```python
from build123d import *

# Parameters (mm, degrees)
SKETCH1_R                    = 69.85
SKETCH1_R_2                  = 55.88
BOSS_EXTRUDE1_DEPTH          = 6.35
BOSS_EXTRUDE2_DEPTH          = 6.35
FILLET1_R                    = 6.35
CIRPATTERN2_COUNT            = 4
FILLET1_OF_CIRPATTERN2_R     = 6.35
F_0_257_DIAMETER_HOLE1_D     = 6.5278
CIRPATTERN1_COUNT            = 4
SKETCH6_R                    = 3.2639
CUT_EXTRUDE1_DEPTH           = 7.3500001
BOSS_EXTRUDE4_DEPTH          = 6.35
FILLET3_R                    = 3.175
F_18_0_1695_DIAMETER_HOLE1_D = 4.3053


with BuildPart() as part:
    # Sketch1 → Boss-Extrude1 (new body)
    with BuildSketch(Plane(origin=(0, 0, 0), x_dir=(1, 0, 0), z_dir=(0, 1, 0))):
        Circle(SKETCH1_R)
        Circle(SKETCH1_R_2, mode=Mode.SUBTRACT)
    extrude(amount=BOSS_EXTRUDE1_DEPTH)

    # Sketch5 → Boss-Extrude2 (add)
    with BuildSketch(Plane(origin=(0, 6.35, 0), x_dir=(1, 0, 0), z_dir=(0, 1, 0))):
        with BuildLine():
            Line((-9.525, 63.5), (9.525, 63.5))
            Line((9.525, 63.5), (9.525, 73.025))
            ThreePointArc((9.525, 73.025), (7.665128061, 77.515128061), (3.175, 79.375))
            Line((3.175, 79.375), (-3.175, 79.375))
            ThreePointArc((-3.175, 79.375), (-7.665128061, 77.515128061), (-9.525, 73.025))
            Line((-9.525, 73.025), (-9.525, 63.5))
        make_face()
    boss_extrude2 = extrude(amount=-BOSS_EXTRUDE2_DEPTH)

    # Fillet1
    fillet1_edges = [part.edges().sort_by_distance(p)[0] for p in [
        (9.525, 3.175, -69.197520729),
        (-9.525, 3.175, -69.197520729),
    ]]
    fillet(fillet1_edges, radius=FILLET1_R)

    # CirPattern2: Boss-Extrude2 ×4 about axis
    cirpattern2_axis = Axis((0, 0, 0), (0, 1, 0))
    for i in range(1, CIRPATTERN2_COUNT):
        add(boss_extrude2.rotate(cirpattern2_axis, i * 360 / CIRPATTERN2_COUNT))

    # Fillet1 of CirPattern2
    fillet1_of_cirpattern2_edges = [part.edges().sort_by_distance(p)[0] for p in [
        (-69.197520729, 3.175, -9.525),
        (-69.197520729, 3.175, 9.525),
        (-9.525, 3.175, 69.197520729),
        (9.525, 3.175, 69.197520729),
        (69.197520729, 3.175, 9.525),
        (69.197520729, 3.175, -9.525),
    ]]
    fillet(fillet1_of_cirpattern2_edges, radius=FILLET1_OF_CIRPATTERN2_R)

    # F (0.257) Diameter Hole1 (through all)
    with Locations(Plane(origin=(0, 6.35, 0), x_dir=(1, 0, 0), z_dir=(0, 1, 0))):
        with Locations((69.85, 0)):
            f_0_257_diameter_hole1 = Hole(F_0_257_DIAMETER_HOLE1_D / 2)

    # CirPattern1: F (0.257) Diameter Hole1 ×4 about axis
    cirpattern1_axis = Axis((0, 0, 0), (0, 1, 0))
    for i in range(1, CIRPATTERN1_COUNT):
        add(f_0_257_diameter_hole1.rotate(cirpattern1_axis, i * 360 / CIRPATTERN1_COUNT), mode=Mode.SUBTRACT)

    # Sketch6 → Cut-Extrude1 (cut, through all)
    with BuildSketch(Plane.XZ):
        with BuildLine():
            Line((-38.749062578, -40.262694263), (-48.149496878, -50.60285022))
            ThreePointArc((-48.149496878, -50.60285022), (-46.98699519, -51.684086361), (-45.800220226, -52.738622728))
            Line((-45.800220226, -52.738622728), (-36.399785925, -42.398466772))
            ThreePointArc((-36.399785925, -42.398466772), (-37.589596152, -41.347269089), (-38.749062578, -40.262694263))
        make_face()
        with BuildLine():
            Line((-36.399785925, -42.398466772), (-45.800220226, -52.738622728))
            ThreePointArc((-45.800220226, -52.738622728), (-31.12686289, -62.531119506), (-14.468129908, -68.335171888))
            add(Edge.make_bspline(
                [(-14.468129908, -68.335171888), (-14.283432872, -68.374276505), (-14.099232, -68.420160929), (-13.915921077, -68.472867364), (-13.733896872, -68.532401891), (-13.553556281, -68.598733654), (-13.249844138, -68.723208999), (-13.125423196, -68.77795645), (-13.002168013, -68.83601258), (-12.88021375, -68.897344809), (-12.759693358, -68.961911786), (-12.355694209, -69.192010649), (-12.079622266, -69.372650227), (-11.814338628, -69.570883737), (-11.56151572, -69.78574391), (-11.322668236, -70.016027336), (-10.782274905, -70.606478562), (-10.496090022, -70.980818219), (-10.244386574, -71.379158998), (-10.029870298, -71.796677829), (-9.854233948, -72.228125174), (-9.660927551, -72.851945664), (-9.610789898, -73.037441883), (-9.567571656, -73.224014536), (-9.531268493, -73.411265552), (-9.501839293, -73.598800252), (-9.479207222, -73.786230121)],
                knots=[0, 0, 0, 0, 0, 0, 0, 0.147493178, 0.147493178, 0.147493178, 0.147493178, 0.147493178, 0.251288922, 0.251288922, 0.251288922, 0.251288922, 0.251288922, 0.500005624, 0.500005624, 0.500005624, 0.500005624, 0.500005624, 0.852506427, 0.852506427, 0.852506427, 0.852506427, 0.852506427, 1, 1, 1, 1, 1, 1, 1], degree=6))
            ThreePointArc((-9.479207222, -73.786230121), (-7.387403633, -77.776647676), (-3.175, -79.375))
            Line((-3.175, -79.375), (3.175, -79.375))
            ThreePointArc((3.175, -79.375), (7.387403633, -77.776647676), (9.479207222, -73.786230121))
            add(Edge.make_bspline(
                [(14.468129908, -68.335171888), (14.283432872, -68.374276505), (14.099232, -68.420160929), (13.915921077, -68.472867364), (13.733896872, -68.532401891), (13.553556281, -68.598733654), (13.249844138, -68.723208999), (13.125423196, -68.77795645), (13.002168013, -68.83601258), (12.88021375, -68.897344809), (12.759693358, -68.961911786), (12.355694209, -69.192010649), (12.079622266, -69.372650227), (11.814338628, -69.570883737), (11.56151572, -69.78574391), (11.322668236, -70.016027336), (10.782274905, -70.606478562), (10.496090022, -70.980818219), (10.244386574, -71.379158998), (10.029870298, -71.796677829), (9.854233948, -72.228125174), (9.660927551, -72.851945664), (9.610789898, -73.037441883), (9.567571656, -73.224014536), (9.531268493, -73.411265552), (9.501839293, -73.598800252), (9.479207222, -73.786230121)],
                knots=[0, 0, 0, 0, 0, 0, 0, 0.147493178, 0.147493178, 0.147493178, 0.147493178, 0.147493178, 0.251288922, 0.251288922, 0.251288922, 0.251288922, 0.251288922, 0.500005624, 0.500005624, 0.500005624, 0.500005624, 0.500005624, 0.852506427, 0.852506427, 0.852506427, 0.852506427, 0.852506427, 1, 1, 1, 1, 1, 1, 1], degree=6))
            ThreePointArc((14.468129908, -68.335171888), (49.391408666, -49.391408666), (68.335171888, -14.468129908))
            add(Edge.make_bspline(
                [(68.335171888, -14.468129908), (68.374276505, -14.283432872), (68.420160929, -14.099232), (68.472867364, -13.915921077), (68.532401891, -13.733896872), (68.598733654, -13.553556281), (68.846403967, -12.949256038), (69.059475497, -12.535015212), (69.310044177, -12.138083802), (69.595960031, -11.763541247), (69.914101744, -11.415952673), (70.50455297, -10.875559342), (70.762813807, -10.667280882), (71.033632627, -10.475600201), (71.315394329, -10.301582166), (71.606347562, -10.146042489), (72.029097801, -9.952540464), (72.154851861, -9.898875057), (72.281748365, -9.84855844), (72.409651228, -9.801620057), (72.53842294, -9.758080416), (72.851945664, -9.660927551), (73.037441883, -9.610789898), (73.224014536, -9.567571656), (73.411265552, -9.531268493), (73.598800252, -9.501839293), (73.786230121, -9.479207222)],
                knots=[0, 0, 0, 0, 0, 0, 0, 0.147493573, 0.147493573, 0.147493573, 0.147493573, 0.147493573, 0.499994376, 0.499994376, 0.499994376, 0.499994376, 0.499994376, 0.748711078, 0.748711078, 0.748711078, 0.748711078, 0.748711078, 0.852506822, 0.852506822, 0.852506822, 0.852506822, 0.852506822, 1, 1, 1, 1, 1, 1, 1], degree=6))
            ThreePointArc((73.786230121, -9.479207222), (77.776647676, -7.387403633), (79.375, -3.175))
            Line((79.375, -3.175), (79.375, 3.175))
            ThreePointArc((79.375, 3.175), (77.776647676, 7.387403633), (73.786230121, 9.479207222))
            add(Edge.make_bspline(
                [(68.335171888, 14.468129908), (68.374276505, 14.283432872), (68.420160929, 14.099232), (68.472867364, 13.915921077), (68.532401891, 13.733896872), (68.598733654, 13.553556281), (68.846403967, 12.949256038), (69.059475497, 12.535015212), (69.310044177, 12.138083802), (69.595960031, 11.763541247), (69.914101744, 11.415952673), (70.50455297, 10.875559342), (70.762813807, 10.667280882), (71.033632627, 10.475600201), (71.315394329, 10.301582166), (71.606347562, 10.146042489), (72.029097801, 9.952540464), (72.154851861, 9.898875057), (72.281748365, 9.84855844), (72.409651228, 9.801620057), (72.53842294, 9.758080416), (72.851945664, 9.660927551), (73.037441883, 9.610789898), (73.224014536, 9.567571656), (73.411265552, 9.531268493), (73.598800252, 9.501839293), (73.786230121, 9.479207222)],
                knots=[0, 0, 0, 0, 0, 0, 0, 0.147493573, 0.147493573, 0.147493573, 0.147493573, 0.147493573, 0.499994376, 0.499994376, 0.499994376, 0.499994376, 0.499994376, 0.748711078, 0.748711078, 0.748711078, 0.748711078, 0.748711078, 0.852506822, 0.852506822, 0.852506822, 0.852506822, 0.852506822, 1, 1, 1, 1, 1, 1, 1], degree=6))
            ThreePointArc((68.335171888, 14.468129908), (60.980316639, 34.064989103), (48.149496878, 50.60285022))
            Line((48.149496878, 50.60285022), (38.749062578, 40.262694263))
            ThreePointArc((38.749062578, 40.262694263), (51.419218279, 21.877805913), (55.88, 0))
            ThreePointArc((55.88, 0), (23.329748847, -50.776935894), (-36.399785925, -42.398466772))
        make_face()
        with Locations((0, -69.85)):
            Circle(SKETCH6_R, mode=Mode.SUBTRACT)
        with Locations((69.85, 0)):
            Circle(SKETCH6_R, mode=Mode.SUBTRACT)
        with BuildLine():
            Line((45.800220226, 52.738622728), (36.399785925, 42.398466772))
            ThreePointArc((36.399785925, 42.398466772), (37.589596152, 41.347269089), (38.749062578, 40.262694263))
            Line((38.749062578, 40.262694263), (48.149496878, 50.60285022))
            ThreePointArc((48.149496878, 50.60285022), (46.98699519, 51.684086361), (45.800220226, 52.738622728))
        make_face()
    extrude(amount=-CUT_EXTRUDE1_DEPTH, mode=Mode.SUBTRACT)

    # Sketch8 → Boss-Extrude4 (add)
    with BuildSketch(Plane(origin=(0, 0, 0), x_dir=(-1, 0, 0), z_dir=(0, -1, 0))):
        with BuildLine():
            Line((47.292152613, 49.659800874), (38.749062578, 40.262694263))
            Line((38.749062578, 40.262694263), (62.241829106, 18.904969177))
            Line((62.241829106, 18.904969177), (66.513374123, 23.603522482))
            ThreePointArc((66.513374123, 23.603522482), (68.15763817, 28.177007956), (66.086365835, 32.573620805))
            Line((66.086365835, 32.573620805), (47.292152613, 49.659800874))
        make_face()
        with BuildLine():
            Line((-36.399785925, -42.398466772), (-44.94287596, -51.795573383))
            Line((-44.94287596, -51.795573383), (-26.148662738, -68.881753452))
            ThreePointArc((-26.148662738, -68.881753452), (-21.575177264, -70.526017499), (-17.178564415, -68.454745164))
            Line((-17.178564415, -68.454745164), (-12.907019398, -63.756191858))
            Line((-12.907019398, -63.756191858), (-36.399785925, -42.398466772))
        make_face()
    extrude(amount=-BOSS_EXTRUDE4_DEPTH)

    # Fillet3
    fillet3_edges = [part.edges().sort_by_distance(p)[0] for p in [
        (-65.95747234, 3.175, -22.992049549),
        (16.622662632, 3.175, 67.843272231),
    ]]
    fillet(fillet3_edges, radius=FILLET3_R)

    # #18 (0.1695) Diameter Hole1 (through all)
    with Locations(Plane(origin=(0, 0, 0), x_dir=(-1, 0, 0), z_dir=(0, -1, 0))):
        with Locations((61.814820818, 27.875067499), (52.417714206, 36.418157534)):
            f_18_0_1695_diameter_hole1 = Hole(F_18_0_1695_DIAMETER_HOLE1_D / 2)

    # Mirror8: #18 (0.1695) Diameter Hole1 across plane
    add(f_18_0_1695_diameter_hole1.mirror(Plane(origin=(0, 0, 0), x_dir=(-0.739929654, 0, 0.672684255), z_dir=(-0.672684255, 0, -0.739929654))), mode=Mode.SUBTRACT)


solid = part.part
```
CAD build for the part. Positions are in the model's coordinates, mm. A direction names the side the tool comes from. Round coordinates to 2 decimals unless told otherwise and drop trailing zeros. Order: outer loops, then holes, each group sorted by start corner. A loop starts at its lowest first (then second) coordinate and runs counter-clockwise, first axis right, second up. Notation, with made-up numbers: (6.25, 79) - (51.25, 79) arc R23 cw to (51.25, 108) - close; hole circle Ø10 at (-4.75, -22.75). An arc over 180 degrees is marked (long way). Use CSV: the item, a comma, the result in double quotes. Start each with the question number.
1) Tool access for faces 5 (the cylindrical face through (-67.5, 3.13, -17.97)), 6 (the flat face through (-45, 0, 38)): list every direction of +Z, -Z, +X, -X, +Y, -Y with a clear straight run to the whole face (end or side of a thin tool).
2) Saw through at C-C (z = 19). List the corners of the cut face in (x, y).
3) Saw through at A-A (z = 0). List the corners of the cut face in (x, y) (3 decimals), and give its area (3 significant figures).
4) Two-plate mould, pull along Z, no slides. Class faces 1 (the cylindrical face through (-68.137, 3.131, -28.468)), 2 (the cylindrical face through (-42.15, 3.13, 36.69)), 3 (the cylindrical face through (21.997, 3.131, 70.532)), 4 (the flat face through (41.166, 3.131, 47.641)): pulls with the +Z half, pulls with the -Z half, needs draft (parallel to the pull), parting line crosses it, or undercut.
5) Wall check: L1, parallel to Z at x = 0, y = 1.5 (3 decimals); L2, parallel to X at y = 5.25, z = 48.5; L3, parallel to Z at x = -43, y = 1.5. Give the ranges that are in metal, low to high. Write a range as [from, to].
6) Saw through at D-D (y = 2.75). Count the separate pieces of the cut face and the enclosed holes in it, and give its area (3 significant figures).
7) Saw through at B-B (x = 0). List the corners of the cut face in (y, z) (3 decimals), and give its area (3 significant figures).
8) Pin check, flat tips, straight feed: pin 1 Ø2.5 at (x, z) = (-52.42, -36.42) entering from +Y; pin 2 Ø1.5 at (x, y) = (-24.5, 4) entering from +Z; pin 3 Ø1 at (x, y) = (-50, 3.5) entering from -Z; pin 4 Ø1 at (y, z) = (5.5, 26.5) entering from -X. Stop position of each tip, or through.
Values follow:
1,face 5,"-X, +Y, -Y"
1,face 6,"+Z, -Z, +X, -X, -Y"
2,outline,"(-67.22, 0) - (-52.55, 0) - (-52.55, 6.35) - (-67.22, 6.35) - close"
3,outline,"(-79.375, 0) - (-73.114, 0) - (-73.114, 6.35) - (-79.375, 6.35) - close; (-66.586, 0) - (-55.88, 0) - (-55.88, 6.35) - (-66.586, 6.35) - close"
3,area,"108 mm2"
4,face 1,"undercut"
4,face 2,"undercut"
4,face 3,"pulls with the +Z half"
4,face 4,"pulls with the -Z half"
5,L1,"z = [55.88, 66.586], [73.114, 79.375]"
5,L2,"x = [-50.27, -27.75], [27.75, 41.95]"
5,L3,"z = [-44.94, -35.69], [35.69, 55.05]"
6,separate pieces,"1"
6,enclosed holes,"6"
6,area,"3,050 mm2"
7,outline,"(0, 55.88) - (6.35, 55.88) - (6.35, 66.586) - (0, 66.586) - close; (0, 73.114) - (6.35, 73.114) - (6.35, 79.375) - (0, 79.375) - close"
7,area,"108 mm2"
8,pin 1,"passes through"
8,pin 2,"stops at z = 65.69"
8,pin 3,"stops at z = -49.28"
8,pin 4,"stops at x = -64.83"
